Can you work these out from the model? Positions are in its coordinate system, mm. Face numbers are marked on the shaded views. A direction names the side the tool comes from. Give positions to 0.01 mm unless a question says otherwise; leave off trailing zeros. Order: outer loops, then holes, each group sorted by start corner. A loop starts at its lowest first (then second) coordinate and runs counter-clockwise, first axis right, second up.
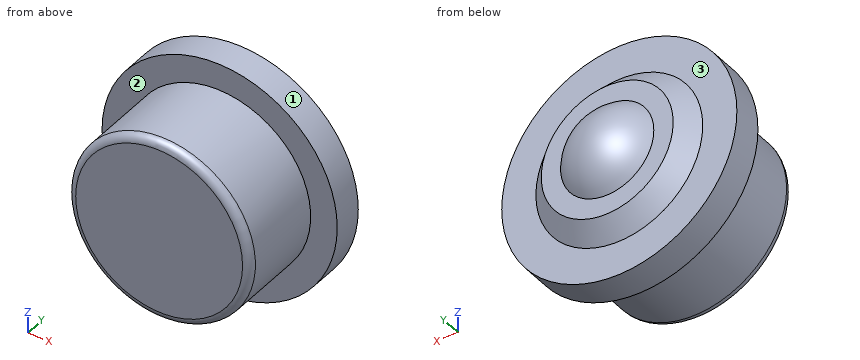
```python
from build123d import *

# Parameters (mm, degrees)
FILLET1_R = 1


with BuildPart() as part:
    # Esquisse1 → Révolution1 (revolve)
    with BuildSketch(Plane.XY):
        with BuildLine():
            Line((-12, -2), (-15.5, -2))
            Line((-15.5, -2), (-15.5, 2))
            Line((-15.5, 2), (-11, 2))
            Line((-11, 2), (-8.7, 4.3))
            Line((-8.7, 4.3), (-6.144916598, 4.3))
            ThreePointArc((-6.144916598, 4.3), (-3.464101615, 6.652067348), (0, 7.5))
            Line((0, 7.5), (0, -13.5))
            Line((0, -13.5), (-12, -13.5))
            Line((-12, -13.5), (-12, -12))
            Line((-12, -12), (-12, -2))
        make_face()
    revolve(axis=Axis((0, 7.5, 0), (0, -1, 0)))

    # Fillet1
    fillet1_edges = [part.edges().sort_by_distance(p)[0] for p in [
        (12, -13.5, 0),
    ]]
    fillet(fillet1_edges, radius=FILLET1_R)


solid = part.part
```
1) Suppose I cut it at C-C (y = -1.5). Please give me the cut outline in (x, z), and give its area (3 significant figures).
2) Suppose I cut it at D-D (x = -13.5). Please give me the cut outline in (y, z), and give its area (3 significant figures).
3) I'm going to push flat-ended pins straight in: pin 1 Ø6 at (x, z) = (10, -6.5) entering from -Y; pin 2 Ø5 at (y, z) = (-11, 3.5) entering from -X; pin 3 Ø4 at (y, z) = (-4.5, -5.5) entering from +X; pin 4 Ø1 at (y, z) = (-11, -2.5) entering from +X. Where does each tip first touch, or does it pass through?
4) If I drill on line 1 (Y direction, x = -8.5, z = 10.5); line 2 (Y direction, x = 8, z = 1); line 3 (X direction, y = -4.25, z = -4), over which ranges is the centre line in solid material (lowest first)?
5) Suppose I cut it at A-A (z = 0). Please give me the cut outline in (x, y).
6) Which directions (+Z, -Z, +X, -X, +Y, -Y) give clear straight access to the entire face, cutting with the end or side of a thin tool? Please do the marked faces 1, 2 and 3.
7) Suppose I cut it at B-B (x = 0). Please give me the cut outline in (y, z).
Results:
1. outline: circle Ø31 at (0, 0)
1. area: 755 mm2
2. outline: (-2, -7.62) - (2, -7.62) - (2, 7.62) - (-2, 7.62) - close
2. area: 60.9 mm2
3. pin 1: stops at y = -13.5
3. pin 2: stops at x = -11.96
3. pin 3: stops at x = 11.48
3. pin 4: stops at x = 11.83
4. line 1: y = -2 to 2
4. line 2: y = -13.5 to 4.3
4. line 3: x = -11.31 to 11.31
5. outline: (-15.5, -2) - (-12, -2) - (-12, -12.5) arc R1 ccw to (-11, -13.5) - (11, -13.5) arc R1 ccw to (12, -12.5) - (12, -2) - (15.5, -2) - (15.5, 2) - (11, 2) - (8.7, 4.3) - (6.14, 4.3) arc R7.5 ccw to (-6.14, 4.3) - (-8.7, 4.3) - (-11, 2) - (-15.5, 2) - close
6. face 1: +Y, -Y
6. face 2: -Y
6. face 3: +Y
7. outline: (-13.5, -11) arc R1 ccw to (-12.5, -12) - (-2, -12) - (-2, -15.5) - (2, -15.5) - (2, -11) - (4.3, -8.7) - (4.3, -6.14) arc R7.5 ccw to (4.3, 6.14) - (4.3, 8.7) - (2, 11) - (2, 15.5) - (-2, 15.5) - (-2, 12) - (-12.5, 12) arc R1 ccw to (-13.5, 11) - close
